Build history of the part. All positions in model axes, mm. A direction names the side the tool comes from. Coordinates: 2 decimals unless noted, no trailing zeros. Order: outer loops, then holes, each group sorted by start corner. A loop starts at its lowest first (then second) coordinate and runs counter-clockwise, first axis right, second up. Notation, with made-up numbers: (-25.5, -33.75) - (6.5, -33.75) arc R28 cw to (6.5, 1.25) - close; hole circle Ø11 at (88, 23.25). An arc over 180 degrees is marked (long way). One line per item, written item: value.
from build123d import *

# Parameters (mm, degrees)
EXTRUDE1_DEPTH     = 6.35
SKETCH2_R          = 3.175
CUT_EXTRUDE1_DEPTH = 7.35
SKETCH3_R          = 1.609646759
CUT_EXTRUDE2_DEPTH = 6.35


with BuildPart() as part:
    # Sketch1 → Extrude1 (new body)
    with BuildSketch(Plane.XY):
        Polygon((-19.501167272, 6.290815989), (-9.976167272, 6.290815989), (-9.976167272, -9.584184011), (5.898832728, -9.584184011), (5.898832728, -19.109184011), (-19.501167272, -19.109184011), align=None)
    extrude(amount=EXTRUDE1_DEPTH)

    # Sketch2 → Cut-Extrude1 (cut, through all)
    with BuildSketch(Plane.XY.offset(6.35)):
        with Locations((1.136332728, -14.346684011)):
            Circle(SKETCH2_R)
    extrude(amount=-CUT_EXTRUDE1_DEPTH, mode=Mode.SUBTRACT)

    # Sketch3 → Cut-Extrude2 (cut)
    with BuildSketch(Plane.ZY.offset(19.501167272)):
        with Locations((3.175, -6.409184011)):
            Circle(SKETCH3_R)
    extrude(amount=-CUT_EXTRUDE2_DEPTH, mode=Mode.SUBTRACT)


solid = part.part
1. Band-saw the part on A-A, the plane x = 2.75. Give the cut face in (y, z).
Values found:
outline: (-19.11, 0) - (-17.08, 0) - (-17.08, 6.35) - (-19.11, 6.35) - close; (-11.61, 0) - (-9.58, 0) - (-9.58, 6.35) - (-11.61, 6.35) - close
2. Two-plate mould, pull along X, no slides. Class faces 1 (the face through (0.448, -17.446, 3.219)), 2 (the face through (-7, -19.109, 3)), 3 (the face through (-13.151, -6, 3)): pulls with the +X half, pulls with the -X half, needs draft (parallel to the pull), parting line crosses it, or undercut.
Values found:
face 1: undercut
face 2: needs draft
face 3: pulls with the -X half
3. Probe line 1 along X through (y, z) = (-6, 5); line 2 along Y through (x, z) = (-5.5, 3.25); line 3 along Y through (x, z) = (-14.25, 2). List the from-to ranges inside material, lowest first.
Values found:
line 1: x = -19.5 to -9.98
line 2: y = -19.11 to -9.58
line 3: y = -19.11 to -7.51, -5.31 to 6.29
4. Flat gauge pins, fed straight in: P1, Ø3, axis at x = 0.5, z = 3, coming from the +Y side; P2, Ø1.6, axis at y = -6, z = 3, coming from the -X side; P3, Ø3, axis at y = -6.41, z = 3.18, coming from the +X side. Where does each tip first touch, or does it go through?
Values found:
P1: stops at y = -9.58
P2: stops at x = -13.15
P3: stops at x = -9.98
5. Band-saw the part on C-C, the plane z = 3.25. Give the cut face in (x, y) (3 decimals), and give its area (3 significant figures).
Values found:
outline: (-19.501, -19.109) - (5.899, -19.109) - (5.899, -9.584) - (-9.976, -9.584) - (-9.976, 6.291) - (-19.501, 6.291) - (-19.501, -4.801) - (-13.151, -4.801) - (-13.151, -8.017) - (-19.501, -8.017) - close; hole circle Ø6.35 at (1.136, -14.347)
area: 341 mm2
6. 3-axis set-ups, long thin cutter, end or side, ignore diameter. For faces 4 (the face through (-9.976, -2, 3)), 5 (the face through (-12, -9, 0)), 6 (the face through (-16.371, -7.837, 3.918)): which of +Z, -Z, +X, -X, +Y, -Y reach the whole face in a straight line?
Values found:
face 4: +Z, -Z, +X, +Y
face 5: -Z, +X, -X, +Y, -Y
face 6: -X
7. Band-saw the part on D-D, the plane x = -16.25. Give the cut face in (y, z) (3 decimals), and give its area (3 significant figures).
Values found:
outline: (-19.109, 0) - (6.291, 0) - (6.291, 6.35) - (-19.109, 6.35) - close; hole circle Ø3.219 at (-6.409, 3.175)
area: 153 mm2
8. Band-saw the part on B-B, the plane y = -12.25. Give the cut face in (x, z).
Values found:
outline: (-19.5, 0) - (-1.25, 0) - (-1.25, 6.35) - (-19.5, 6.35) - close; (3.52, 0) - (5.9, 0) - (5.9, 6.35) - (3.52, 6.35) - close
